Work out the finished part from the listing and answer in its coordinate system (mm). Coordinates: 2 decimals unless noted, no trailing zeros. Write each loop counter-clockwise with the first axis right and the second up, starting at its lowest first coordinate (ties: lowest second). Pieces come first, ordered by that corner, then holes. Notation, with made-up numbers: M 61.25,-4 L 84.25,-4 A20 cw 84.25,28 Z; hole C -20.75,-19 d6. An arc over 180 degrees is marked long. Answer as CSV lines item,"result". Start each with the question number.
(1) Find the intervals of material crossed by L1, parallel to X at y = 0, z = 1.7; L2, parallel to Y at x = 45.6, z = 3.25; L3, parallel to Y at x = 21.5, z = 3.3, in increasing order. Write a range as [from, to].
(2) A cutting plane is placed at A-A on x = 24.5. Give the vertices of the cut face in (y, z).
(3) Flat-ended cylindrical pins translate along their axes: P1, Ø1.5, axis at y = 3, z = 1.5, coming from the -X side; P2, Ø3, axis at y = -8.5, z = 2.5, coming from the +X side; P3, Ø1.5, axis at y = 2.5, z = 2.5, coming from the +X side. Find the tip coordinate at first contact, or state that the pin passes through.
(4) A cutting plane is placed at D-D on z = 3.4. Count the separate pieces of the cut face and the enclosed holes in it, then the cut area to 3 significant figures.
(5) A cutting plane is placed at C-C on y = 5. Give the vertices of the cut face in (x, z).
(6) A cutting plane is placed at B-B on x = 45.6. Give the vertices of the cut face in (y, z), then the cut area to 3 significant figures.
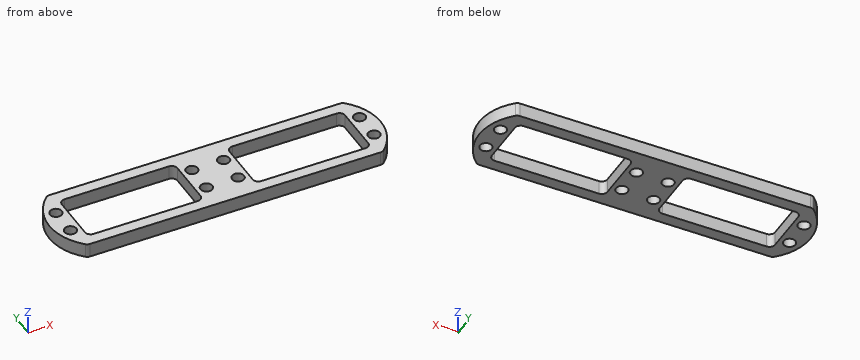
from build123d import *

# Parameters (mm, degrees)
EXTRUSION1_DEPTH        = 5
ESQUISSE2_R             = 2.1
ENL_V_MAT_EXTRU_1_DEPTH = 100.61551084


with BuildPart() as part:
    # Esquisse1 → Extrusion1 (new body)
    with BuildSketch(Plane.XY):
        with BuildLine():
            Line((-11.324751653, 14), (91.324751653, 14))
            ThreePointArc((91.324751653, 14), (92.063300599, 13.858640755), (92.697448823, 13.454545455))
            ThreePointArc((92.697448823, 13.454545455), (98.5, 0), (92.697448823, -13.454545455))
            ThreePointArc((92.697448823, -13.454545455), (92.063300599, -13.858640755), (91.324751653, -14))
            Line((91.324751653, -14), (-11.324751653, -14))
            ThreePointArc((-11.324751653, -14), (-12.063300599, -13.858640755), (-12.697448823, -13.454545455))
            ThreePointArc((-12.697448823, -13.454545455), (-18.5, 0), (-12.697448823, 13.454545455))
            ThreePointArc((-12.697448823, 13.454545455), (-12.063300599, 13.858640755), (-11.324751653, 14))
        make_face()
        with BuildLine():
            Line((51.215395011, 9.95), (88, 9.95))
            ThreePointArc((88, 9.95), (89.414213562, 9.364213562), (90, 7.95))
            Line((90, 7.95), (90, -7.95))
            ThreePointArc((90, -7.95), (89.414213562, -9.364213562), (88, -9.95))
            Line((88, -9.95), (51.215395011, -9.95))
            ThreePointArc((51.215395011, -9.95), (49.801181448, -9.364213562), (49.215395011, -7.95))
            Line((49.215395011, -7.95), (49.215395011, 7.95))
            ThreePointArc((49.215395011, 7.95), (49.801181448, 9.364213562), (51.215395011, 9.95))
        make_face(mode=Mode.SUBTRACT)
        with BuildLine():
            Line((-8, 9.95), (28.8, 9.95))
            ThreePointArc((28.8, 9.95), (30.214213562, 9.364213562), (30.8, 7.95))
            Line((30.8, 7.95), (30.8, -7.95))
            ThreePointArc((30.8, -7.95), (30.214213562, -9.364213562), (28.8, -9.95))
            Line((28.8, -9.95), (-8, -9.95))
            ThreePointArc((-8, -9.95), (-9.414213562, -9.364213562), (-10, -7.95))
            Line((-10, -7.95), (-10, 7.95))
            ThreePointArc((-10, 7.95), (-9.414213562, 9.364213562), (-8, 9.95))
        make_face(mode=Mode.SUBTRACT)
    extrude(amount=EXTRUSION1_DEPTH)

    # Esquisse2 → Enlèv. mat.-Extru.1 (cut, through all)
    with BuildSketch(Plane.XY):
        with Locations((-13.6, 5)):
            Circle(ESQUISSE2_R)
        with Locations((45.6, -5)):
            Circle(ESQUISSE2_R)
        with Locations((34.4, 5)):
            Circle(ESQUISSE2_R)
        with Locations((-13.6, -5)):
            Circle(ESQUISSE2_R)
        with Locations((93.6, 5)):
            Circle(ESQUISSE2_R)
        with Locations((93.6, -5)):
            Circle(ESQUISSE2_R)
        with Locations((45.6, 5)):
            Circle(ESQUISSE2_R)
        with Locations((34.4, -5)):
            Circle(ESQUISSE2_R)
    extrude(amount=ENL_V_MAT_EXTRU_1_DEPTH, mode=Mode.SUBTRACT)


solid = part.part
Here are the results:
1,L1,"x = [-18.5, -10], [30.8, 49.22], [90, 98.5]"
1,L2,"y = [-14, -7.1], [-2.9, 2.9], [7.1, 14]"
1,L3,"y = [-14, -9.95], [9.95, 14]"
2,outline,"M -14,0 L -9.95,0 L -9.95,5 L -14,5 Z; M 9.95,0 L 14,0 L 14,5 L 9.95,5 Z"
3,P1,"stops at x = -18.36"
3,P2,"stops at x = 97.12"
3,P3,"stops at x = 98.42"
4,separate pieces,"1"
4,enclosed holes,"10"
4,area,"1,440 mm^2"
5,outline,"M -17.81,0 L -15.7,0 L -15.7,5 L -17.81,5 Z; M -11.5,0 L -10,0 L -10,5 L -11.5,5 Z; M 30.8,0 L 32.3,0 L 32.3,5 L 30.8,5 Z; M 36.5,0 L 43.5,0 L 43.5,5 L 36.5,5 Z; M 47.7,0 L 49.22,0 L 49.22,5 L 47.7,5 Z; M 90,0 L 91.5,0 L 91.5,5 L 90,5 Z; M 95.7,0 L 97.81,0 L 97.81,5 L 95.7,5 Z"
6,outline,"M -14,0 L -7.1,0 L -7.1,5 L -14,5 Z; M -2.9,0 L 2.9,0 L 2.9,5 L -2.9,5 Z; M 7.1,0 L 14,0 L 14,5 L 7.1,5 Z"
6,area,"98.0 mm^2"
